Design review of the part shown in the three views and the two pictorial views. Dimensions are in mm from the part's minimum x, y and z. Round coordinates to 2 decimals unless told otherwise and drop trailing zeros. Loops run counter-clockwise (first coordinate to the right, second up) from the corner with the lowest first, then second, coordinate; pieces in that order, holes last. Notation, with made-up numbers: (-35, -14) -> (-17, -14) arc R22 cw to (-17, 16) -> close; hole circle Ø7 at (7, 16.25). An arc over 180 degrees is marked (long way). Use a Markdown table: item, result. Add a question column.
1) Wall thickness on probe 1 along X at (y, z) = (14.25, 178.5): over which ranges is the line inside the solid? List them lowest first.
2) Insertion check: pin 1 (4 mm diameter, centred on y = 2.5, z = 363.5, fed in from -X); pin 2 (9.5 mm diameter, centred on x = 18.5, y = 6, fed in from +Z); pin 3 (1.5 mm diameter, centred on y = 2.5, z = 175, fed in from +X). Each pin has a flat end and moves straight along its axis. Give the tip position at first contact, or say it passes through.
3) Consider section B-B on z = 275. Give the boundary of the cut face in (x, y), plus the area to 3 significant figures.
4) Consider section A-A on y = 10. Give the boundary of the cut face in (x, z), plus the area to 3 significant figures.
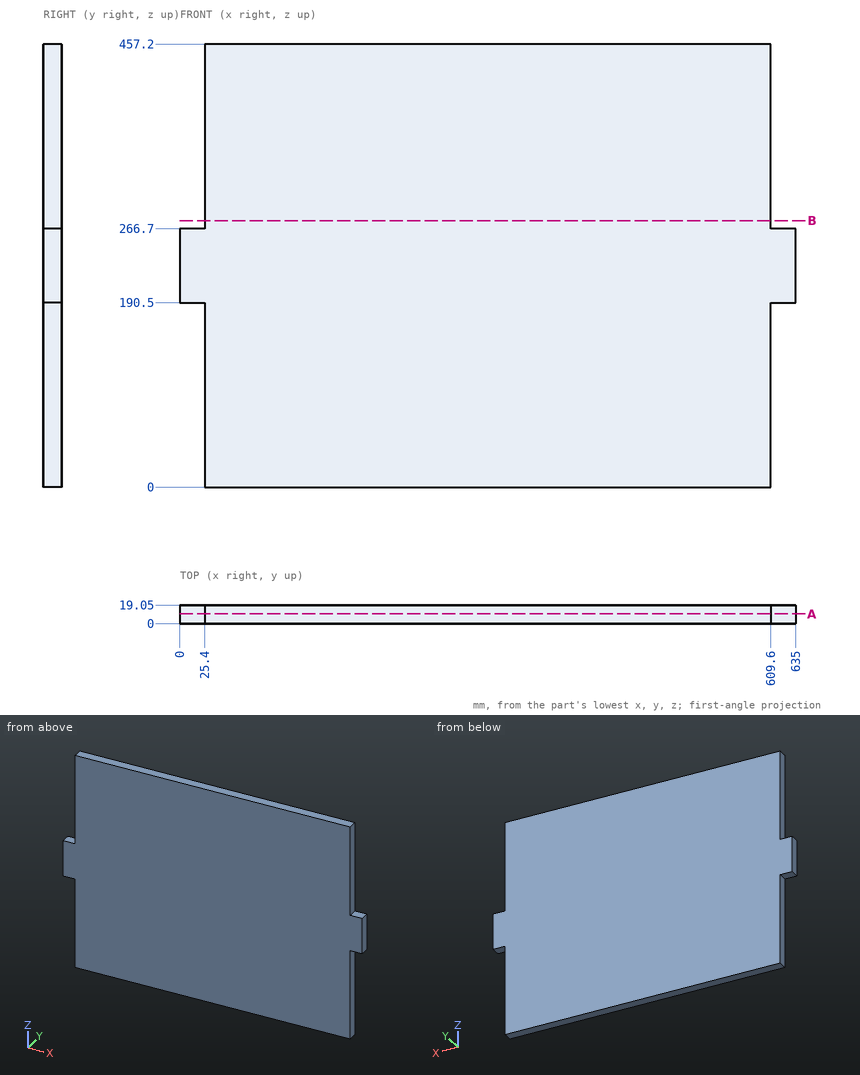
Result set:
| question | item | result |
|---|---|---|
| 1 | probe 1 | 25.4 to 609.6 |
| 2 | pin 1 | x = 25.4 |
| 2 | pin 2 | z = 266.7 |
| 2 | pin 3 | x = 609.6 |
| 3 | outline | (25.4, 0) -> (609.6, 0) -> (609.6, 19.05) -> (25.4, 19.05) -> close |
| 3 | area | 11,100 mm2 |
| 4 | outline | (0, 190.5) -> (25.4, 190.5) -> (25.4, 0) -> (609.6, 0) -> (609.6, 190.5) -> (635, 190.5) -> (635, 266.7) -> (609.6, 266.7) -> (609.6, 457.2) -> (25.4, 457.2) -> (25.4, 266.7) -> (0, 266.7) -> close |
| 4 | area | 271,000 mm2 |
